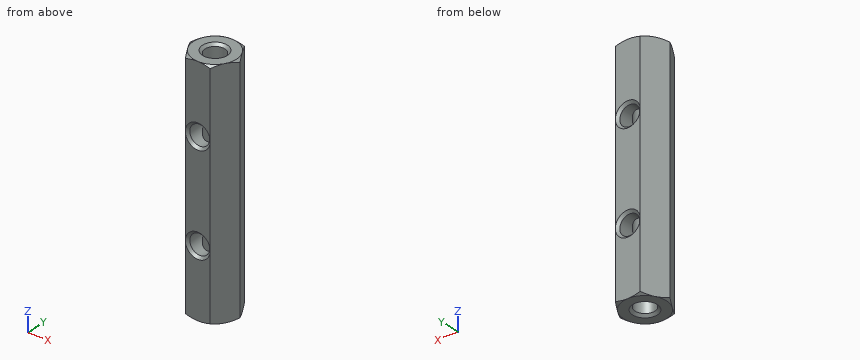
```python
from build123d import *

# Parameters (mm, degrees)
EXTRUDE_1_DEPTH          = 9.5
SKETCH_2_OUTSIDE_W       = 79.862
SKETCH_2_OUTSIDE_H       = 79.326
SKETCH_2_OUTSIDE_R       = 1.732050808
CUT_EXTRUDE_1_DEPTH      = 20.183326093
CUT_EXTRUDE_1_DRAFT      = -60
HOLE_WIZARD_M2_1_D       = 1.6
HOLE_WIZARD_M2_2_D       = 1.6
MIRROR_1_COPY_1_SKETCH_W = 79.862
MIRROR_1_COPY_1_SKETCH_H = 79.326
MIRROR_1_COPY_1_SKETCH_R = 1.732050808
MIRROR_1_COPY_1_DEPTH    = 20.183326093
MIRROR_1_COPY_1_DRAFT    = -60
CHAMFER_1_SIZE           = 0.2


with BuildPart() as part:
    # 草图1 → 凸台-拉伸1 (new, symmetric)
    with BuildSketch(Plane.XY):
        Polygon((2, 0), (1, 1.732050808), (-1, 1.732050808), (-2, 0), (-1, -1.732050808), (1, -1.732050808), align=None)
    extrude(amount=EXTRUDE_1_DEPTH, both=True)


with BuildPart() as cut_extrude_1_tool:
    # 草图2 outside → 切除-拉伸1 (with draft: the straight prism first)
    with BuildSketch(Plane.XY.offset(9.5)):
        Rectangle(SKETCH_2_OUTSIDE_W, SKETCH_2_OUTSIDE_H)
        Circle(SKETCH_2_OUTSIDE_R, mode=Mode.SUBTRACT)
    extrude(amount=-CUT_EXTRUDE_1_DEPTH)
    # 切除-拉伸1: the draft: its side faces are tilted about the plane it starts from
    cut_extrude_1_sides = [cut_extrude_1_tool.faces().sort_by_distance(p)[0] for p in [
        (0, -39.663, -0.591663047),
        (39.931, 0, -0.591663047),
        (0, 39.663, -0.591663047),
        (-39.931, 0, -0.591663047),
        (-1.732050808, 0, -0.591663047),
    ]]
    draft(cut_extrude_1_sides, Plane.XY.offset(9.5), CUT_EXTRUDE_1_DRAFT)


with BuildPart() as part_1:
    add(part.part)

    # 切除-拉伸1: cut by cut_extrude_1_tool
    add(cut_extrude_1_tool.part, mode=Mode.SUBTRACT)

    # M2 螺纹孔1 (through all)
    with Locations(Plane.XY.offset(9.5)):
        with Locations((0, 0)):
            hole_wizard_m2_1 = Hole(HOLE_WIZARD_M2_1_D / 2)

    # M2 螺纹孔2 (through all)
    with Locations(Plane(origin=(0, 1.732050808, 0), x_dir=(1, 0, 0), z_dir=(0, 1, 0))):
        with Locations((0, -4)):
            hole_wizard_m2_2 = Hole(HOLE_WIZARD_M2_2_D / 2)

    # 镜向1: M2 螺纹孔1, M2 螺纹孔2 across plane
    add(hole_wizard_m2_1.mirror(Plane.XY), mode=Mode.SUBTRACT)
    add(hole_wizard_m2_2.mirror(Plane.XY), mode=Mode.SUBTRACT)


with BuildPart() as mirror_1_copy_1_tool:
    # 镜向1 copy 1 sketch → 镜向1 copy 1 (with draft: the straight prism first)
    with BuildSketch(Plane(origin=(0, 0, -9.5), x_dir=(1, 0, 0), z_dir=(0, 0, -1))):
        Rectangle(MIRROR_1_COPY_1_SKETCH_W, MIRROR_1_COPY_1_SKETCH_H)
        Circle(MIRROR_1_COPY_1_SKETCH_R, mode=Mode.SUBTRACT)
    extrude(amount=-MIRROR_1_COPY_1_DEPTH)
    # 镜向1 copy 1: the draft: its side faces are tilted about the plane it starts from
    mirror_1_copy_1_sides = [mirror_1_copy_1_tool.faces().sort_by_distance(p)[0] for p in [
        (0, -39.663, 0.591663047),
        (39.931, 0, 0.591663047),
        (0, 39.663, 0.591663047),
        (-39.931, 0, 0.591663047),
        (-1.732050808, 0, 0.591663047),
    ]]
    draft(mirror_1_copy_1_sides, Plane(origin=(0, 0, -9.5), x_dir=(1, 0, 0), z_dir=(0, 0, -1)), MIRROR_1_COPY_1_DRAFT)


with BuildPart() as part_2:
    add(part_1.part)

    # 镜向1 copy 1: cut by mirror_1_copy_1_tool
    add(mirror_1_copy_1_tool.part, mode=Mode.SUBTRACT)

    # 倒角1
    chamfer_1_edges = [part_2.edges().sort_by_distance(p)[0] for p in [
        (0.8, -1.732050808, -4),
        (0.8, 1.732050808, -4),
        (0.8, 0, 9.5),
        (0.8, 0, -9.5),
        (0.8, -1.732050808, 4),
        (0.8, 1.732050808, 4),
    ]]
    chamfer(chamfer_1_edges, length=CHAMFER_1_SIZE - 0.0001)  # a hair under: the kernel refuses the full size


solid = part_2.part
```
Input: part model. Units: mm. Frame: model coordinates. Give positions to 0.01 mm unless a question says otherwise; leave off trailing zeros. Write each loop counter-clockwise with the first axis right and the second up, starting at its lowest first coordinate (ties: lowest second). Pieces come first, ordered by that corner, then holes. Notation, with made-up numbers: (5, -36) - (60, -36) arc R31 ccw to (60, -7) - close; hole circle Ø1 at (12, 17). An arc over 180 degrees is marked (long way). Write item = value, one per line. Start each with the question number.
1. Section query A-A, the plane z = 1.5. Output: boundary loops of the cut face in (x, y).
2. First-contact query: pin 1 Ø1.3 at (x, z) = (0, 4) entering from +Y; pin 2 Ø1.5 at (x, y) = (1.5, -1) entering from +Z. Flat tips, straight axial feed; report the tip coordinate or a pass-through.
3. Section query B-B, the plane x = -0.45. Count the separate pieces of the cut face and the enclosed holes in it, then the cut area to 3 significant figures.
4. Ray query, L1, parallel to Z at x = -0.1, y = -1.35; L2, parallel to Z at x = -0.7, y = -0.8; L3, parallel to X at y = -0.8, z = 3.5. Return the intervals inside material, ascending.
Check sheet entries:
q1.outline = (-2, 0) - (-1, -1.73) - (1, -1.73) - (2, 0) - (1, 1.73) - (-1, 1.73) - close; hole circle Ø1.6 at (0, 0)
q2.pin_1 = through
q2.pin_2 = 9.5
q3.separate_pieces = 6
q3.enclosed_holes = 0
q3.area = 34.7 mm2
q4.L1 = -9.5 to -4.79, -3.21 to 3.21, 4.79 to 9.5
q4.L2 = -9.5 to -4.39, -3.61 to 3.61, 4.39 to 9.5
q4.L3 = -1.54 to -0.62, 0.62 to 1.54
